Input: part model. Units: mm. Frame: model coordinates. Face numbers are marked on the shaded views. A direction names the side the tool comes from. Coordinates: 2 decimals unless noted, no trailing zeros. Order: outer loops, then holes, each group sorted by start corner. A loop starts at its lowest first (then second) coordinate and runs counter-clockwise, first axis right, second up. Notation, with made-up numbers: M -15,34 L 30,34 A7 cw 30,44 Z; hole C -12,19 d3. An arc over 180 degrees is marked long. Answer in a Markdown table with one row per item.
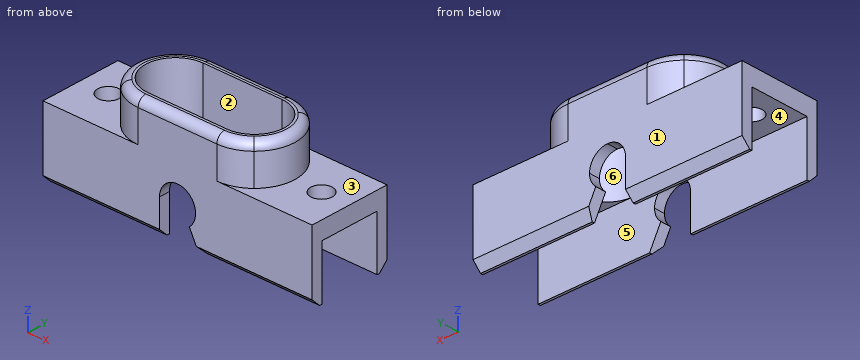
from build123d import *

# Parameters (mm, degrees)
F1_DEPTH = 6.1341
F2_DEPTH = 11.0744
F0_R     = 1.651
F3_DEPTH = 2.7432
F5_DEPTH = 12.5232
F6_SIZE  = 1.27
F7_R     = 1.27


with BuildPart() as f1:
    # F0 (on Top) → F1 (new body)
    with BuildSketch(Plane.XY):
        with BuildLine():
            Line((14.75105, 1.651), (10.514501, 1.651))
            ThreePointArc((10.514501, 1.651), (12.477608, 0.427333), (14.75105, 0))
            Line((14.75105, 0), (20.8534, 0))
            Line((20.8534, 0), (26.95575, 0))
            ThreePointArc((26.95575, 0), (29.229192, 0.427333), (31.192299, 1.651))
            Line((31.192299, 1.651), (26.95575, 1.651))
            Line((26.95575, 1.651), (20.8534, 1.651))
            Line((20.8534, 1.651), (14.75105, 1.651))
        make_face()
        with BuildLine():
            Line((14.75105, 10.8712), (10.514501, 10.8712))
            ThreePointArc((10.514501, 10.8712), (8.48995, 6.2611), (10.514501, 1.651))
            Line((10.514501, 1.651), (14.75105, 1.651))
            ThreePointArc((14.75105, 1.651), (10.14095, 6.2611), (14.75105, 10.8712))
        make_face()
        with BuildLine():
            Line((20.8534, 12.5222), (14.75105, 12.5222))
            ThreePointArc((14.75105, 12.5222), (12.477608, 12.094867), (10.514501, 10.8712))
            Line((10.514501, 10.8712), (14.75105, 10.8712))
            Line((14.75105, 10.8712), (20.8534, 10.8712))
            Line((20.8534, 10.8712), (26.95575, 10.8712))
            Line((26.95575, 10.8712), (31.192299, 10.8712))
            ThreePointArc((31.192299, 10.8712), (29.229192, 12.094867), (26.95575, 12.5222))
            Line((26.95575, 12.5222), (20.8534, 12.5222))
        make_face()
        with BuildLine():
            ThreePointArc((31.192299, 1.651), (33.21685, 6.2611), (31.192299, 10.8712))
            Line((31.192299, 10.8712), (26.95575, 10.8712))
            ThreePointArc((26.95575, 10.8712), (31.56585, 6.2611), (26.95575, 1.651))
            Line((26.95575, 1.651), (31.192299, 1.651))
        make_face()
    extrude(amount=F1_DEPTH)

    # F0 (on Top) → F2 (join)
    with BuildSketch(Plane.XY):
        with BuildLine():
            Line((10.514501, 1.651), (0, 1.651))
            Line((0, 1.651), (0, 0))
            Line((0, 0), (14.75105, 0))
            ThreePointArc((14.75105, 0), (12.477608, 0.427333), (10.514501, 1.651))
        make_face()
        with BuildLine():
            Line((14.75105, 1.651), (10.514501, 1.651))
            ThreePointArc((10.514501, 1.651), (12.477608, 0.427333), (14.75105, 0))
            Line((14.75105, 0), (20.8534, 0))
            Line((20.8534, 0), (26.95575, 0))
            ThreePointArc((26.95575, 0), (29.229192, 0.427333), (31.192299, 1.651))
            Line((31.192299, 1.651), (26.95575, 1.651))
            Line((26.95575, 1.651), (20.8534, 1.651))
            Line((20.8534, 1.651), (14.75105, 1.651))
        make_face()
        with BuildLine():
            Line((41.7068, 1.651), (31.192299, 1.651))
            ThreePointArc((31.192299, 1.651), (29.229192, 0.427333), (26.95575, 0))
            Line((26.95575, 0), (41.7068, 0))
            Line((41.7068, 0), (41.7068, 1.651))
        make_face()
        with BuildLine():
            Line((14.75105, 12.5222), (0, 12.5222))
            Line((0, 12.5222), (0, 10.8712))
            Line((0, 10.8712), (10.514501, 10.8712))
            ThreePointArc((10.514501, 10.8712), (12.477608, 12.094867), (14.75105, 12.5222))
        make_face()
        with BuildLine():
            Line((20.8534, 12.5222), (14.75105, 12.5222))
            ThreePointArc((14.75105, 12.5222), (12.477608, 12.094867), (10.514501, 10.8712))
            Line((10.514501, 10.8712), (14.75105, 10.8712))
            Line((14.75105, 10.8712), (20.8534, 10.8712))
            Line((20.8534, 10.8712), (26.95575, 10.8712))
            Line((26.95575, 10.8712), (31.192299, 10.8712))
            ThreePointArc((31.192299, 10.8712), (29.229192, 12.094867), (26.95575, 12.5222))
            Line((26.95575, 12.5222), (20.8534, 12.5222))
        make_face()
        with BuildLine():
            Line((41.7068, 12.5222), (26.95575, 12.5222))
            ThreePointArc((26.95575, 12.5222), (29.229192, 12.094867), (31.192299, 10.8712))
            Line((31.192299, 10.8712), (41.7068, 10.8712))
            Line((41.7068, 10.8712), (41.7068, 12.5222))
        make_face()
    extrude(amount=-F2_DEPTH)

    # F0 (on Top) → F3 (join)
    with BuildSketch(Plane.XY):
        with BuildLine():
            Line((14.75105, 10.8712), (10.514501, 10.8712))
            ThreePointArc((10.514501, 10.8712), (8.48995, 6.2611), (10.514501, 1.651))
            Line((10.514501, 1.651), (14.75105, 1.651))
            ThreePointArc((14.75105, 1.651), (10.14095, 6.2611), (14.75105, 10.8712))
        make_face()
        with BuildLine():
            Line((10.514501, 10.8712), (0, 10.8712))
            Line((0, 10.8712), (0, 1.651))
            Line((0, 1.651), (10.514501, 1.651))
            ThreePointArc((10.514501, 1.651), (8.48995, 6.2611), (10.514501, 10.8712))
        make_face()
        with Locations((4.3434, 6.2611)):
            Circle(F0_R, mode=Mode.SUBTRACT)
        with BuildLine():
            ThreePointArc((31.192299, 1.651), (33.21685, 6.2611), (31.192299, 10.8712))
            Line((31.192299, 10.8712), (26.95575, 10.8712))
            ThreePointArc((26.95575, 10.8712), (31.56585, 6.2611), (26.95575, 1.651))
            Line((26.95575, 1.651), (31.192299, 1.651))
        make_face()
        with BuildLine():
            Line((41.7068, 10.8712), (31.192299, 10.8712))
            ThreePointArc((31.192299, 10.8712), (33.21685, 6.2611), (31.192299, 1.651))
            Line((31.192299, 1.651), (41.7068, 1.651))
            Line((41.7068, 1.651), (41.7068, 10.8712))
        make_face()
        with Locations((37.3634, 6.2611)):
            Circle(F0_R, mode=Mode.SUBTRACT)
    extrude(amount=-F3_DEPTH)

    # F4 (on Front) → F5 (cut, through all)
    with BuildSketch(Plane.XZ):
        with BuildLine():
            ThreePointArc((23.6474, -5.5372), (22.829056, -3.561544), (20.8534, -2.7432))
            ThreePointArc((20.8534, -2.7432), (18.877744, -3.561544), (18.0594, -5.5372))
            Line((18.0594, -5.5372), (22.677582, -7.653517))
            ThreePointArc((22.677582, -7.653517), (23.3934, -6.701174), (23.6474, -5.5372))
        make_face()
        with BuildLine():
            Line((22.677582, -7.653517), (18.0594, -5.5372))
            ThreePointArc((18.0594, -5.5372), (19.689426, -8.0772), (22.677582, -7.653517))
        make_face()
        with BuildLine():
            Line((18.0594, -5.5372), (18.0594, -11.0744))
            Line((18.0594, -11.0744), (24.4094, -11.0744))
            Line((24.4094, -11.0744), (22.677582, -7.653517))
            ThreePointArc((22.677582, -7.653517), (19.689426, -8.0772), (18.0594, -5.5372))
        make_face()
    extrude(amount=-F5_DEPTH, mode=Mode.SUBTRACT)

    # F6
    f6_edges = [f1.edges().sort_by_distance(p)[0] for p in [
        (33.0581, 0, -11.0744),
        (9.0297, 0, -11.0744),
        (33.0581, 12.5222, -11.0744),
        (9.0297, 12.5222, -11.0744),
    ]]
    chamfer(f6_edges, length=F6_SIZE)

    # F7
    f7_edges = [f1.edges().sort_by_distance(p)[0] for p in [
        (33.21685, 6.2611, 6.1341),
        (20.8534, 12.5222, 6.1341),
    ]]
    fillet(f7_edges, radius=F7_R)


solid = f1.part
1) Cut plane A-A, the plane x = 15.5. Output: boundary loops of the cut face in (y, z).
Resolved:
| item | result |
|---|---|
| outline | M 0,-9.8 L 1.27,-11.07 L 1.65,-11.07 L 1.65,6.13 L 1.27,6.13 A1.27 ccw 0,4.86 Z; M 10.87,-11.07 L 11.25,-11.07 L 12.52,-9.8 L 12.52,4.86 A1.27 ccw 11.25,6.13 L 10.87,6.13 Z |
2) Cut plane C-C, the plane z = -4.25. Output: boundary loops of the cut face in (x, y).
Resolved:
| item | result |
|---|---|
| outline | M 0,0 L 18.37,0 L 18.37,1.65 L 0,1.65 Z; M 0,10.87 L 18.37,10.87 L 18.37,12.52 L 0,12.52 Z; M 23.33,0 L 41.71,0 L 41.71,1.65 L 23.33,1.65 Z; M 23.33,10.87 L 41.71,10.87 L 41.71,12.52 L 23.33,12.52 Z |
3) Cut plane B-B, the plane z = 0.5. Output: boundary loops of the cut face in (x, y).
Resolved:
| item | result |
|---|---|
| outline | M 10.51,1.65 A6.26 ccw 14.75,0 L 26.96,0 A6.26 ccw 31.19,1.65 A6.26 ccw 31.19,10.87 A6.26 ccw 26.96,12.52 L 14.75,12.52 A6.26 ccw 10.51,10.87 A6.26 ccw Z; hole M 14.75,1.65 L 26.96,1.65 A4.61 ccw 26.96,10.87 L 14.75,10.87 A4.61 ccw Z |
4) Material intervals for probe 1 along Y at (x, z) = (27, 4.25); probe 2 along X at (y, z) = (0.75, -5.75); probe 3 along Y at (x, z) = (28, 4), sorted ascending.
Resolved:
| item | result |
|---|---|
| probe 1 | y = 0 to 1.65, 10.87 to 12.52 |
| probe 2 | x = 0 to 18.06, 23.64 to 41.71 |
| probe 3 | y = 0.09 to 1.77, 10.75 to 12.43 |
5) Cut plane D-D, the plane x = 7. Output: boundary loops of the cut face in (y, z), and give its area (3 significant figures).
Resolved:
| item | result |
|---|---|
| outline | M 0,-9.8 L 1.27,-11.07 L 1.65,-11.07 L 1.65,-2.74 L 10.87,-2.74 L 10.87,-11.07 L 11.25,-11.07 L 12.52,-9.8 L 12.52,0 L 0,0 Z |
| area | 60.2 mm2 |
6) Reachability of the marked faces 4, 5 and 6 from +Z, -Z, +X, -X, +Y, -Y: full face, straight path, thin tool, end or side. Return the list, or none.
Resolved:
| item | result |
|---|---|
| face 4 | -Z, +X, -X |
| face 5 | -Z |
| face 6 | +Z, -Z |
7) Mould query, pull axis Y, two halves, no side actions, for the marked faces 1, 2 and 3. Classes: +Y half, -Y half, draft (parallel to the pull), parting line (faces both ways), or undercut.
Resolved:
| item | result |
|---|---|
| face 1 | +Y half |
| face 2 | undercut |
| face 3 | draft |
8) Contact query for flat-ended pins moving along their axis: pin 1 (6 mm diameter, centred on x = 14, y = 5.5, fed in from +Z); pin 2 (4 mm diameter, centred on x = 37.36, y = 6.26, fed in from +Z); pin 3 (3 mm diameter, centred on x = 35.5, y = 4.5, fed in from -Z). Output: stop coordinate, or through.
Resolved:
| item | result |
|---|---|
| pin 1 | passes through |
| pin 2 | stops at z = 0 |
| pin 3 | stops at z = -2.74 |
